from build123d import *

# Parameters (mm, degrees)
SKETCH1_W           = 106.814150222
SKETCH1_H           = 8
EXTRUDE1_DEPTH      = 5
EXTRUDE2_DEPTH      = 5
LPATTERN1_COUNT     = 34
LPATTERN1_PITCH     = 3.141592654
SKETCH_2_W          = 106.814150222
SKETCH_2_H          = 5
EXTRUDE_1_DEPTH     = 4.25
SKETCH_3_W          = 5
SKETCH_3_H          = 17.759873191
CUT_EXTRUDE_1_DEPTH = 6.814150222
SKETCH_4_R          = 1.15
CUT_EXTRUDE_2_DEPTH = 101.87151481
SKETCH_5_W          = 30
SKETCH_5_H          = 20
EXTRUDE_2_DEPTH     = 5
SKETCH_6_R          = 1.65
CUT_EXTRUDE_3_DEPTH = 13


with BuildPart() as part:
    # Sketch1 → Extrude1 (new body)
    with BuildSketch(Plane.XY):
        with Locations((53.407075111, -4)):
            Rectangle(SKETCH1_W, SKETCH1_H)
    extrude(amount=EXTRUDE1_DEPTH)

    # Sketch2 → Extrude2 (add)
    with BuildSketch(Plane.XY.offset(5)):
        Polygon((0, 0), (0.818933027, 2.25), (1.661788885, 2.25), (2.480721912, 0), align=None)
    extrude2 = extrude(amount=-EXTRUDE2_DEPTH)

    # LPattern1: Extrude2 ×34
    with Locations(*[(i * LPATTERN1_PITCH, 0, 0) for i in range(1, LPATTERN1_COUNT)]):
        add(extrude2)

    # 草图2 → 凸台-拉伸1 (add)
    with BuildSketch(Plane.XZ.offset(8)):
        with Locations((53.407075111, 2.5)):
            Rectangle(SKETCH_2_W, SKETCH_2_H)
    extrude(amount=EXTRUDE_1_DEPTH)

    # 草图3 → 切除-拉伸1 (cut)
    with BuildSketch(Plane(origin=(106.814150222, 0, 0), x_dir=(0, 0, -1), z_dir=(1, 0, 0))):
        with Locations((-2.5, -3.370063404)):
            Rectangle(SKETCH_3_W, SKETCH_3_H)
    extrude(amount=-CUT_EXTRUDE_1_DEPTH, mode=Mode.SUBTRACT)

    # 草图4 → 切除-拉伸2 (cut, through all)
    with BuildSketch(Plane.XY.offset(5)):
        with Locations((5, -8.75)):
            Circle(SKETCH_4_R)
        with Locations((20, -8.75)):
            Circle(SKETCH_4_R)
        with Locations((35, -8.75)):
            Circle(SKETCH_4_R)
        with Locations((50, -8.75)):
            Circle(SKETCH_4_R)
        with Locations((65, -8.75)):
            Circle(SKETCH_4_R)
        with Locations((80, -8.75)):
            Circle(SKETCH_4_R)
        with Locations((95, -8.75)):
            Circle(SKETCH_4_R)
    extrude(amount=-CUT_EXTRUDE_2_DEPTH, mode=Mode.SUBTRACT)

    # 草图5 → 凸台-拉伸2 (add)
    with BuildSketch(Plane.XY.offset(5)):
        with Locations((15, -22.25)):
            Rectangle(SKETCH_5_W, SKETCH_5_H)
    extrude(amount=-EXTRUDE_2_DEPTH)

    # 草图6 → 切除-拉伸3 (cut)
    with BuildSketch(Plane.XY.offset(5)):
        with Locations((25, -27.25)):
            Circle(SKETCH_6_R)
        with Locations((5, -27.25)):
            Circle(SKETCH_6_R)
    extrude(amount=-CUT_EXTRUDE_3_DEPTH, mode=Mode.SUBTRACT)


solid = part.part
Can you work these out from the model? Positions are in its coordinate system, mm. A direction names the side the tool comes from. Coordinates: 2 decimals unless noted, no trailing zeros. Write each loop counter-clockwise with the first axis right and the second up, starting at its lowest first coordinate (ties: lowest second). Pieces come first, ordered by that corner, then holes.
Q1. Imagine slicing it at A-A, the plane y = -27.25. List the corners of the cut face in (x, z) for me.
Results found:
outline: (0, 0) - (3.35, 0) - (3.35, 5) - (0, 5) - close; (6.65, 0) - (23.35, 0) - (23.35, 5) - (6.65, 5) - close; (26.65, 0) - (30, 0) - (30, 5) - (26.65, 5) - close
Q2. If we mould it in two halves opening along X, with no side actions, what happens to faces 1 (the face through (72.66, 1.11, 2.54)), 2 (the face through (38, -11, 0)), 3 (the face through (30, -22, 3))? For each: +X half, -X half, draft (parallel to the pull), parting line (faces both ways), or undercut.
Results found:
face 1: undercut
face 2: draft
face 3: +X half
Q3. Please list where these lines run through material, in increasing order: L1, parallel to Y at x = 80, z = 1.3; L2, parallel to Y at x = 20, z = 3.1; L3, parallel to X at y = -29.5, z = 2.8.
Results found:
L1: y = -12.25 to -9.9, -7.6 to 2.25
L2: y = -32.25 to -9.9, -7.6 to 2.25
L3: x = 0 to 30
Q4. Imagine slicing it at D-D, the plane y = -22. List the corners of the cut face in (x, z) for me.
Results found:
outline: (0, 0) - (30, 0) - (30, 5) - (0, 5) - close
Q5. For P1, Ø2, axis at x = 20, y = -8.75, coming from the -Z side; P2, Ø2, axis at y = -22, z = 1, coming from the +X side, each with a flat end and sliding along its axis, tell me the tip position at first contact or that it passes through.
Results found:
P1: passes through
P2: stops at x = 30
Q6. Which directions (+Z, -Z, +X, -X, +Y, -Y) give clear straight access to the entire face, cutting with the end or side of a thin tool? Please do faces 4 (the face through (79.09, -9.45, 2.54)), 5 (the face through (78.944, 1.109, 2.535)).
Results found:
face 4: +Z, -Z
face 5: +Z, -Z, +Y
Q7. Imagine slicing it at B-B, the plane y = -8.75. Count the separate pieces of the cut face and the enclosed holes in it, plus the area to 4 significant figures.
Results found:
separate pieces: 8
enclosed holes: 0
area: 419.5 mm2
